Work out the finished part from the listing and answer in its coordinate system (mm). A direction names the side the tool comes from. Coordinates: 2 decimals unless noted, no trailing zeros. Order: outer loops, then holes, each group sorted by start corner. A loop starts at its lowest first (then second) coordinate and runs counter-clockwise, first axis right, second up. Notation, with made-up numbers: (22.5, -26) -> (42.5, -26) arc R15 ccw to (42.5, -4) -> close; hole circle Ø1 at (-2.5, 86). An arc over 180 degrees is marked (long way). Write item = value, one per line. Start each with the question number.
Q1. The part is cut by section C-C, the plane y = 22. Determine the outline of the cut face in (x, z), plus the area to 3 significant figures.
Q2. For a pull along Z with two mould halves and no side action, classify faces 4 (the flat face through (-1, 33, -59.399)), 5 (the flat face through (1, 39, -62.932)), 6 (the flat face through (0, 5, 45)) as +Z half, -Z half, draft (parallel to the pull), parting line (faces both ways), or undercut.
Q3. The part is cut by section D-D, the plane z = -40.5. Determine the outline of the cut face in (x, y).
Q4. Straight lines are drawn through the part: L1, parallel to Y at x = -13, z = -48.5; L2, parallel to Y at x = 7, z = -24; L3, parallel to X at y = 6.5, z = 8. For each, find the intervals that lie inside material, in ascending order. Write a range as from..to.
Q5. Which of the six approach directions +Z, -Z, +X, -X, +Y, -Y give full straight-line access (tool end or side, diameter ignored) to faces 1 (the flat face through (-48, 10, 18)), 2 (the flat face through (-0.7, 34.857, -38.052)), 3 (the flat face through (1, 80.018, -8))?
Q6. The part is cut by section A-A, the plane z = 8.5. Determine the outline of the cut face in (x, y).
Q7. The part is cut by section B-B, the plane x = 38.5. Determine the outline of the cut face in (y, z), plus the area to 3 significant figures.
```python
from build123d import *

# Parameters (mm, degrees)
SKETCH_2_W               = 5
SKETCH_2_H               = 90
EXTRUDE_1_DEPTH          = 10
EXTRUDE_1_2_DEPTH        = 10
SKETCH_2_W_2             = 50
EXTRUDE_1_3_DEPTH        = 10
EXTRUDE_5_DEPTH          = 50
SKETCH_5_W               = 107.932472338
SKETCH_5_H               = 8
EXTRUDE_6_DEPTH          = 50
CUT_EXTRUDE_1_DEPTH      = 114.416886857
CUT_EXTRUDE_1_DEPTH_BACK = 114.416886857
FILLET_1_R               = 2
FILLET_2_R               = 2


with BuildPart() as part:
    # Sketch 2 → Extrude 1 (new body)
    with BuildSketch(Plane(origin=(0, 0, 0), x_dir=(1, 0, 0), z_dir=(0, 1, 0))):
        with Locations((-47.5, 0)):
            Rectangle(SKETCH_2_W, SKETCH_2_H)
    extrude(amount=EXTRUDE_1_DEPTH)



with BuildPart() as body_2:
    # Sketch 2 → Extrude 1 2 (new body)
    with BuildSketch(Plane(origin=(0, 0, 0), x_dir=(1, 0, 0), z_dir=(0, 1, 0))):
        with Locations((47.5, 0)):
            Rectangle(SKETCH_2_W, SKETCH_2_H)
    extrude(amount=EXTRUDE_1_2_DEPTH)


with BuildPart() as body_3:
    # Sketch 2 → Extrude 1 3 (new body)
    with BuildSketch(Plane(origin=(0, 0, 0), x_dir=(1, 0, 0), z_dir=(0, 1, 0))):
        Rectangle(SKETCH_2_W_2, SKETCH_2_H)
    extrude(amount=EXTRUDE_1_3_DEPTH)


with BuildPart() as part_1:
    add(part.part)

    add(body_2.part)  # Extrude 5 merges body 2

    add(body_3.part)  # Extrude 5 merges body 3
    # Sketch 3 → Extrude 5 (add, symmetric)
    with BuildSketch(Plane(origin=(0, 0, 0), x_dir=(0, 0, -1), z_dir=(1, 0, 0))):
        Polygon((62.932472338, 75), (0, 0), (45, 0), (62.932472338, 0), align=None)
    extrude(amount=EXTRUDE_5_DEPTH, both=True)

    # Sketch 5 → Extrude 6 (add, symmetric)
    with BuildSketch(Plane(origin=(0, 0, 0), x_dir=(0, 0, -1), z_dir=(1, 0, 0))):
        with Locations((8.966236169, 76.018086392)):
            Rectangle(SKETCH_5_W, SKETCH_5_H)
    extrude(amount=EXTRUDE_6_DEPTH, both=True)

    # Sketch 6 → Cut-Extrude 1 (cut, two sides: drawn at the far end of the back side and taken through both)
    with BuildSketch(Plane(origin=(0, 0, 0), x_dir=(0, 0, -1), z_dir=(1, 0, 0)).offset(-CUT_EXTRUDE_1_DEPTH_BACK)):
        Polygon((18.156116312, 10), (59.398505248, 61.526811336), (59.398505248, 10), align=None)
    extrude(amount=CUT_EXTRUDE_1_DEPTH + CUT_EXTRUDE_1_DEPTH_BACK, mode=Mode.SUBTRACT)

    # Fillet 1
    fillet_1_edges = [part_1.edges().sort_by_distance(p)[0] for p in [
        (0, 61.526811336, -59.398505248),
        (0, 10, -18.156116312),
    ]]
    fillet(fillet_1_edges, radius=FILLET_1_R)

    # Fillet 2
    fillet_2_edges = [part_1.edges().sort_by_distance(p)[0] for p in [
        (0, 72.018086392, -60.430349729),
    ]]
    fillet(fillet_2_edges, radius=FILLET_2_R)


solid = part_1.part
```
Model answer:
q1.outline = (-50, -62.93) -> (50, -62.93) -> (50, -59.4) -> (-50, -59.4) -> close; (-50, -27.76) -> (50, -27.76) -> (50, -18.46) -> (-50, -18.46) -> close
q1.area = 1,280 mm2
q2.face_4 = undercut
q2.face_5 = -Z half
q2.face_6 = +Z half
q3.outline = (-50, 0) -> (50, 0) -> (50, 10) -> (-50, 10) -> close; (-50, 37.92) -> (50, 37.92) -> (50, 48.27) -> (-50, 48.27) -> close; (-50, 72.02) -> (50, 72.02) -> (50, 80.02) -> (-50, 80.02) -> close
q4.L1 = 0..10, 47.91..57.8, 72.02..80.02
q4.L2 = 0..10, 17.3..28.6, 72.02..80.02
q4.L3 = -50..-45, -25..25, 45..50
q5.face_1 = +Z, +X, -X
q5.face_2 = +X, -X
q5.face_3 = +Z, -Z, +X, -X, +Y
q6.outline = (-50, 0) -> (-45, 0) -> (-45, 10) -> (-50, 10) -> close; (-50, 72.02) -> (50, 72.02) -> (50, 80.02) -> (-50, 80.02) -> close; (-25, 0) -> (25, 0) -> (25, 10) -> (-25, 10) -> close; (45, 0) -> (50, 0) -> (50, 10) -> (45, 10) -> close
q7.outline = (0, -62.93) -> (80.02, -62.93) -> (80.02, 45) -> (72.02, 45) -> (72.02, -56.14) arc R2 cw to (68.73, -57.67) -> (0, 0) -> close; hole (10, -59.4) -> (55.83, -59.4) arc R2 ccw to (57.08, -55.84) -> (13.25, -20.76) arc R2 ccw to (10, -22.32) -> close
q7.area = 2,170 mm2
